```python
from build123d import *

# Parameters (mm, degrees)
SKETCH1_W               = 60.079999982
SKETCH1_H               = 43.079999946
BOSS_EXTRUDE1_DEPTH     = 18.039999988
SHELL1_T                = -2.54
SKETCH2_W               = 114.3
SKETCH2_H               = 43.439999988
BOSS_EXTRUDE2_DEPTH     = 2.54
FILLET1_R               = 5.08
CUT_EXTRUDE1_DEPTH      = 109.11455079
CUT_EXTRUDE1_DEPTH_BACK = 109.11455079
SKETCH3_R               = 1.984375
SKETCH5_W               = 44.45
SKETCH5_H               = 15.499999988
CUT_EXTRUDE2_DEPTH      = 96.606517007
SKETCH6_W               = 37
SKETCH6_H               = 15.499999988
CUT_EXTRUDE3_DEPTH      = 110.54640155


with BuildPart() as part:
    # Sketch1 → Boss-Extrude1 (new body)
    with BuildSketch(Plane(origin=(0, 0, 0), x_dir=(1, 0, 0), z_dir=(0, 1, 0))):
        with Locations((0, 21.539999973)):
            Rectangle(SKETCH1_W, SKETCH1_H)
    extrude(amount=BOSS_EXTRUDE1_DEPTH)

    # Shell1
    shell1_openings = [part.faces().sort_by_distance(p)[0] for p in [
        (0, 18.039999988, -21.539999973),
    ]]
    offset(amount=SHELL1_T, openings=shell1_openings, kind=Kind.INTERSECTION)

    # Sketch2 → Boss-Extrude2 (add)
    with BuildSketch(Plane(origin=(30.039999991, 0, 0), x_dir=(0, 0, -1), z_dir=(1, 0, 0))):
        with Locations((21.539999973, 21.719999994)):
            Rectangle(SKETCH2_W, SKETCH2_H)
    extrude(amount=BOSS_EXTRUDE2_DEPTH)

    # Fillet1
    # the kernel refuses this fillet: 5.08 mm, written as the material it adds along each edge
    with BuildSketch(Plane(origin=(30.039999991, 18.039999988, -43.079999946), x_dir=(0, 1, 0), z_dir=(0, 0, 1))) as fillet1_piece_1_section:
        with BuildLine():
            CenterArc((FILLET1_R, FILLET1_R), FILLET1_R, 180, 90)
            Line((0, FILLET1_R), (0, 0))
            Line((0, 0), (FILLET1_R, 0))
        make_face()
    fillet1_piece_1 = extrude(amount=43.079999946, mode=Mode.PRIVATE)
    fillet1_piece_1 = split(fillet1_piece_1, bisect_by=Plane(origin=(29.204889828, 19.336009893, -40.539999946), z_dir=(0, 0, -1)), keep=Keep.TOP, mode=Mode.PRIVATE)
    fillet1_piece_1 = split(fillet1_piece_1, bisect_by=Plane(origin=(27.499999991, 19.336009893, -41.809999946), z_dir=(1, 0, 0)), keep=Keep.TOP, mode=Mode.PRIVATE)
    add(fillet1_piece_1)
    with BuildSketch(Plane(origin=(30.039999991, 18.039999988, -43.079999946), x_dir=(0, 1, 0), z_dir=(0, 0, 1))) as fillet1_piece_2_section:
        with BuildLine():
            CenterArc((FILLET1_R, FILLET1_R), FILLET1_R, 180, 90)
            Line((0, FILLET1_R), (0, 0))
            Line((0, 0), (FILLET1_R, 0))
        make_face()
    fillet1_piece_2 = extrude(amount=43.079999946, mode=Mode.PRIVATE)
    fillet1_piece_2 = split(fillet1_piece_2, bisect_by=Plane(origin=(26.670686006, 18.161962567, -40.539999946), z_dir=(0, 0, -1)), keep=Keep.TOP, mode=Mode.PRIVATE)
    fillet1_piece_2 = split(fillet1_piece_2, bisect_by=Plane(origin=(27.499999991, 18.161962567, -41.809999946), z_dir=(-1, 0, 0)), keep=Keep.TOP, mode=Mode.PRIVATE)
    add(fillet1_piece_2)
    with BuildSketch(Plane(origin=(30.039999991, 18.039999988, -43.079999946), x_dir=(0, 1, 0), z_dir=(0, 0, 1))) as fillet1_piece_3_section:
        with BuildLine():
            CenterArc((FILLET1_R, FILLET1_R), FILLET1_R, 180, 90)
            Line((0, FILLET1_R), (0, 0))
            Line((0, 0), (FILLET1_R, 0))
        make_face()
    fillet1_piece_3 = extrude(amount=43.079999946, mode=Mode.PRIVATE)
    fillet1_piece_3 = split(fillet1_piece_3, bisect_by=Plane(origin=(29.204889828, 19.336009893, -40.539999946), z_dir=(0, 0, 1)), keep=Keep.TOP, mode=Mode.PRIVATE)
    fillet1_piece_3 = split(fillet1_piece_3, bisect_by=Plane(origin=(29.204889828, 19.336009893, -2.54), z_dir=(0, 0, -1)), keep=Keep.TOP, mode=Mode.PRIVATE)
    fillet1_piece_3 = split(fillet1_piece_3, bisect_by=Plane(origin=(27.499999991, 19.336009893, -21.539999973), z_dir=(1, 0, 0)), keep=Keep.TOP, mode=Mode.PRIVATE)
    add(fillet1_piece_3)
    with BuildSketch(Plane(origin=(30.039999991, 18.039999988, -43.079999946), x_dir=(0, 1, 0), z_dir=(0, 0, 1))) as fillet1_piece_4_section:
        with BuildLine():
            CenterArc((FILLET1_R, FILLET1_R), FILLET1_R, 180, 90)
            Line((0, FILLET1_R), (0, 0))
            Line((0, 0), (FILLET1_R, 0))
        make_face()
    fillet1_piece_4 = extrude(amount=43.079999946, mode=Mode.PRIVATE)
    fillet1_piece_4 = split(fillet1_piece_4, bisect_by=Plane(origin=(29.204889828, 19.336009893, -2.54), z_dir=(0, 0, 1)), keep=Keep.TOP, mode=Mode.PRIVATE)
    fillet1_piece_4 = split(fillet1_piece_4, bisect_by=Plane(origin=(27.499999991, 19.336009893, -1.27), z_dir=(1, 0, 0)), keep=Keep.TOP, mode=Mode.PRIVATE)
    add(fillet1_piece_4)
    with BuildSketch(Plane(origin=(30.039999991, 18.039999988, -43.079999946), x_dir=(0, 1, 0), z_dir=(0, 0, 1))) as fillet1_piece_5_section:
        with BuildLine():
            CenterArc((FILLET1_R, FILLET1_R), FILLET1_R, 180, 90)
            Line((0, FILLET1_R), (0, 0))
            Line((0, 0), (FILLET1_R, 0))
        make_face()
    fillet1_piece_5 = extrude(amount=43.079999946, mode=Mode.PRIVATE)
    fillet1_piece_5 = split(fillet1_piece_5, bisect_by=Plane(origin=(26.670686006, 18.161962567, -2.54), z_dir=(0, 0, 1)), keep=Keep.TOP, mode=Mode.PRIVATE)
    fillet1_piece_5 = split(fillet1_piece_5, bisect_by=Plane(origin=(27.499999991, 18.161962567, -1.27), z_dir=(-1, 0, 0)), keep=Keep.TOP, mode=Mode.PRIVATE)
    add(fillet1_piece_5)

    # Sketch3 → Cut-Extrude1 (cut, two sides: drawn at the far end of the back side and taken through both)
    with BuildSketch(Plane.ZY.offset(-30.039999991).offset(-CUT_EXTRUDE1_DEPTH_BACK)):
        with Locations((-72.339999973, 37.089999988)):
            Circle(SKETCH3_R)
        with Locations((29.260000027, 37.089999988)):
            Circle(SKETCH3_R)
    extrude(amount=CUT_EXTRUDE1_DEPTH + CUT_EXTRUDE1_DEPTH_BACK, mode=Mode.SUBTRACT)

    # Sketch5 → Cut-Extrude2 (cut, through all)
    with BuildSketch(Plane.XY):
        with Locations((0, 10.289999994)):
            Rectangle(SKETCH5_W, SKETCH5_H)
    extrude(amount=-CUT_EXTRUDE2_DEPTH, mode=Mode.SUBTRACT)

    # Sketch6 → Cut-Extrude3 (cut, through all)
    with BuildSketch(Plane.ZY.offset(30.039999991)):
        with Locations((-21.539999973, 10.289999994)):
            Rectangle(SKETCH6_W, SKETCH6_H)
    extrude(amount=-CUT_EXTRUDE3_DEPTH, mode=Mode.SUBTRACT)


solid = part.part
```
Part model, mm, in its own coordinate system. A direction names the side the tool comes from. Round coordinates to 2 decimals unless told otherwise and drop trailing zeros. Loops run counter-clockwise (first coordinate to the right, second up) from the corner with the lowest first, then second, coordinate; pieces in that order, holes last.
1. Two-plate mould, pull along Z, no slides. Class faces 1 (the face through (31, 21, -78.69)), 2 (the face through (24, 18.04, -1)), 3 (the face through (-29, 10, -40.04)): pulls with the +Z half, pulls with the -Z half, needs draft (parallel to the pull), parting line crosses it, or undercut.
Solutions:
face 1: pulls with the -Z half
face 2: needs draft
face 3: undercut
2. 3-axis set-ups, long thin cutter, end or side, ignore diameter. For faces 4 (the face through (-22.225, 10, -1)), 5 (the face through (-29, 10, -3.04)), 6 (the face through (-25, 10, -40.54)), 7 (the face through (30.04, 27, -21)), 8 (the face through (24, 18.04, -42)): which of +Z, -Z, +X, -X, +Y, -Y reach the whole face in a straight line?
Solutions:
face 4: +Z, -Z, +Y
face 5: +X, -X, +Y
face 6: +Y
face 7: -X, +Y
face 8: +Z, -Z, -X, +Y
3. Slice it at D-D (z = -7). Give the cut face in (x, y).
Solutions:
outline: (-30.04, 0) - (32.58, 0) - (32.58, 2.54) - (-30.04, 2.54) - close; (27.5, 18.04) - (32.58, 18.04) - (32.58, 43.44) - (30.04, 43.44) - (30.04, 23.12) arc R5.08 cw to (27.5, 18.72) - close
4. Drill centre lines: line 1 along Z through (x, y) = (31, 37); line 2 along X through (y, z) = (16, -2) (3 decimals); line 3 along Y through (x, z) = (30.6, 29.26). Where is each one in solid material? Low to high.
Solutions:
line 1: z = -78.69 to -74.32, -70.36 to 27.28, 31.24 to 35.61
line 2: x = -30.04 to -22.225, 22.225 to 32.58
line 3: y = 0 to 35.11, 39.07 to 43.44
5. Flat gauge pins, fed straight in: pin 1 (5 mm diameter, centred on y = 18, z = 6, fed in from -X); pin 2 (4 mm diameter, centred on x = -26, y = 14, fed in from +Z); pin 3 (6 mm diameter, centred on x = -24.5, y = 9, fed in from -Z). Where does each tip first touch, or does it go through?
Solutions:
pin 1: stops at x = 30.04
pin 2: stops at z = 0
pin 3: stops at z = -43.08
6. Slice it at C-C (y = 37.09). Give the cut face in (x, z).
Solutions:
outline: (30.04, -78.69) - (32.58, -78.69) - (32.58, -74.32) - (30.04, -74.32) - close; (30.04, -70.36) - (32.58, -70.36) - (32.58, 27.28) - (30.04, 27.28) - close; (30.04, 31.24) - (32.58, 31.24) - (32.58, 35.61) - (30.04, 35.61) - close
7. Slice it at B-B (y = 6.5). Give the cut face in (x, z) (3 decimals).
Solutions:
outline: (-30.04, -43.08) - (-22.225, -43.08) - (-22.225, -40.54) - (-27.5, -40.54) - (-27.5, -40.04) - (-30.04, -40.04) - close; (-30.04, -3.04) - (-27.5, -3.04) - (-27.5, -2.54) - (-22.225, -2.54) - (-22.225, 0) - (-30.04, 0) - close; (22.225, -43.08) - (30.04, -43.08) - (30.04, -78.69) - (32.58, -78.69) - (32.58, -40.04) - (27.5, -40.04) - (27.5, -40.54) - (22.225, -40.54) - close; (22.225, -2.54) - (27.5, -2.54) - (27.5, -3.04) - (32.58, -3.04) - (32.58, 35.61) - (30.04, 35.61) - (30.04, 0) - (22.225, 0) - close
8. Slice it at A-A (z = 29.26). Give the cut face in (x, y).
Solutions:
outline: (30.04, 0) - (32.58, 0) - (32.58, 35.11) - (30.04, 35.11) - close; (30.04, 39.07) - (32.58, 39.07) - (32.58, 43.44) - (30.04, 43.44) - close
